Read the model definition and answer for the solid it produces. Units are mm, in the model's axes. Round coordinates to 2 decimals unless told otherwise and drop trailing zeros. Order: outer loops, then holes, each group sorted by start corner. A loop starts at its lowest first (then second) coordinate and runs counter-clockwise, first axis right, second up.
from build123d import *
from OCP.BRepFilletAPI import BRepFilletAPI_MakeChamfer

# Parameters (mm, degrees)
SKETCH2_R           = 49.911
SKETCH2_R_2         = 7.62
SKETCH2_R_3         = 9.6266
BOSS_EXTRUDE3_DEPTH = 7.62
SKETCH4_R           = 4.064
CUT_EXTRUDE1_DEPTH  = 71.994931101
SKETCH5_R           = 1.905
SKETCH5_R_2         = 9.6266
CUT_EXTRUDE2_DEPTH  = 71.994931101
CHAMFER1_SIZE       = 2.032
CHAMFER1_SIZE2      = 1.422821718


with BuildPart() as part:
    # Sketch2 → Boss-Extrude3 (new body)
    with BuildSketch(Plane.XY):
        with Locations(Location((0, 0, 0), (0, 0, 180))):
            Circle(SKETCH2_R)
        with Locations(Location((0, 0, 0), (0, 0, 180))):
            Circle(SKETCH2_R_2, mode=Mode.SUBTRACT)
        with Locations(Location((0.005302646, -19.066344944, 0), (0, 0, 180))):
            Circle(SKETCH2_R_3, mode=Mode.SUBTRACT)
        with Locations(Location((18.140112855, -5.903126437, 0), (0, 0, 180))):
            Circle(SKETCH2_R_3, mode=Mode.SUBTRACT)
        with Locations(Location((11.225112662, 15.411761203, 0), (0, 0, 180))):
            Circle(SKETCH2_R_3, mode=Mode.SUBTRACT)
        with Locations(Location((-11.183402698, 15.421867724, 0), (0, 0, 180))):
            Circle(SKETCH2_R_3, mode=Mode.SUBTRACT)
        with Locations(Location((-18.117626635, -5.886773743, 0), (0, 0, 180))):
            Circle(SKETCH2_R_3, mode=Mode.SUBTRACT)
        with Locations(Location((-38.862, 0, 0), (0, 0, 180))):
            Circle(SKETCH2_R_3, mode=Mode.SUBTRACT)
        with Locations(Location((-31.453761301, -22.864504732, 0), (0, 0, 180))):
            Circle(SKETCH2_R_3, mode=Mode.SUBTRACT)
        with Locations(Location((-12.020951612, -37.007824175, 0), (0, 0, 180))):
            Circle(SKETCH2_R_3, mode=Mode.SUBTRACT)
        with Locations(Location((12.013756262, -37.027691016, 0), (0, 0, 180))):
            Circle(SKETCH2_R_3, mode=Mode.SUBTRACT)
        with Locations(Location((31.469920822, -22.916516796, 0), (0, 0, 180))):
            Circle(SKETCH2_R_3, mode=Mode.SUBTRACT)
        with Locations(Location((38.915948498, -0.064290447, 0), (0, 0, 180))):
            Circle(SKETCH2_R_3, mode=Mode.SUBTRACT)
        with Locations(Location((31.507709799, 22.800214285, 0), (0, 0, 180))):
            Circle(SKETCH2_R_3, mode=Mode.SUBTRACT)
        with Locations(Location((12.07490011, 36.943533728, 0), (0, 0, 180))):
            Circle(SKETCH2_R_3, mode=Mode.SUBTRACT)
        with Locations(Location((-11.959807763, 36.963400568, 0), (0, 0, 180))):
            Circle(SKETCH2_R_3, mode=Mode.SUBTRACT)
        with Locations(Location((-31.415972324, 22.852226349, 0), (0, 0, 180))):
            Circle(SKETCH2_R_3, mode=Mode.SUBTRACT)
    extrude(amount=BOSS_EXTRUDE3_DEPTH)

    # Sketch4 → Cut-Extrude1 (cut, through all)
    with BuildSketch(Plane.XY.offset(7.62)):
        with Locations((0, 26.17695394)):
            Circle(SKETCH4_R)
        with Locations((24.895762621, 8.037987129)):
            Circle(SKETCH4_R)
        with Locations((15.337793775, -21.244539145)):
            Circle(SKETCH4_R)
        with Locations((-15.465118457, -21.203168848)):
            Circle(SKETCH4_R)
        with Locations((-24.944396322, 8.104925676)):
            Circle(SKETCH4_R)
    extrude(amount=-CUT_EXTRUDE1_DEPTH, mode=Mode.SUBTRACT)

    # Sketch5 → Cut-Extrude2 (cut, through all)
    with BuildSketch(Plane(origin=(0, 0, 0), x_dir=(-1, 0, 0), z_dir=(0, 0, -1))):
        with Locations((-0.00287222, -45.643800189)):
            Circle(SKETCH5_R)
        with Locations((-0.00287222, -32.960144289)):
            Circle(SKETCH5_R)
        with Locations((12.020951612, -37.007824175)):
            Circle(SKETCH5_R_2)
        with Locations((-43.398142788, -14.092845642)):
            Circle(SKETCH5_R)
        with Locations((-31.335269193, -10.173380418)):
            Circle(SKETCH5_R)
        with Locations((-26.801277951, 36.928290351)):
            Circle(SKETCH5_R)
        with Locations((-19.346012068, 26.666997177)):
            Circle(SKETCH5_R)
        with Locations((26.851419192, 36.910131993)):
            Circle(SKETCH5_R)
        with Locations((19.396153308, 26.648838818)):
            Circle(SKETCH5_R)
        with Locations((43.413744778, -14.122226483)):
            Circle(SKETCH5_R)
        with Locations((31.350871183, -10.20276126)):
            Circle(SKETCH5_R)
    extrude(amount=-CUT_EXTRUDE2_DEPTH, mode=Mode.SUBTRACT)

    # Chamfer1: one chamfer whose edges measure the first distance from different faces: ONE call of the kernel's chamfer builder (chamfer() names one face for all edges)
    chamfer1_edges_1 = [part.edges().sort_by_distance(p)[0] for p in [
        (-4.064, 26.17695394, 0),
    ]]
    chamfer1_side_1 = [part.faces().sort_by_distance(p)[0] for p in [
        (-4.064, 26.17695394, 3.81),
    ]]
    chamfer1_edges_2 = [part.edges().sort_by_distance(p)[0] for p in [
        (20.831762621, 8.037987129, 0),
    ]]
    chamfer1_side_2 = [part.faces().sort_by_distance(p)[0] for p in [
        (20.831762621, 8.037987129, 3.81),
    ]]
    chamfer1_edges_3 = [part.edges().sort_by_distance(p)[0] for p in [
        (11.273793775, -21.244539145, 0),
    ]]
    chamfer1_side_3 = [part.faces().sort_by_distance(p)[0] for p in [
        (11.273793775, -21.244539145, 3.81),
    ]]
    chamfer1_edges_4 = [part.edges().sort_by_distance(p)[0] for p in [
        (-19.529118457, -21.203168848, 0),
    ]]
    chamfer1_side_4 = [part.faces().sort_by_distance(p)[0] for p in [
        (-19.529118457, -21.203168848, 3.81),
    ]]
    chamfer1_edges_5 = [part.edges().sort_by_distance(p)[0] for p in [
        (-29.008396322, 8.104925676, 0),
    ]]
    chamfer1_side_5 = [part.faces().sort_by_distance(p)[0] for p in [
        (-29.008396322, 8.104925676, 3.81),
    ]]
    chamfer1 = BRepFilletAPI_MakeChamfer(part.part.solid().wrapped)
    for e in chamfer1_edges_1:
        chamfer1.Add(CHAMFER1_SIZE, CHAMFER1_SIZE2, e.wrapped, chamfer1_side_1[0].wrapped)  # the first distance lies on this face
    for e in chamfer1_edges_2:
        chamfer1.Add(CHAMFER1_SIZE, CHAMFER1_SIZE2, e.wrapped, chamfer1_side_2[0].wrapped)  # the first distance lies on this face
    for e in chamfer1_edges_3:
        chamfer1.Add(CHAMFER1_SIZE, CHAMFER1_SIZE2, e.wrapped, chamfer1_side_3[0].wrapped)  # the first distance lies on this face
    for e in chamfer1_edges_4:
        chamfer1.Add(CHAMFER1_SIZE, CHAMFER1_SIZE2, e.wrapped, chamfer1_side_4[0].wrapped)  # the first distance lies on this face
    for e in chamfer1_edges_5:
        chamfer1.Add(CHAMFER1_SIZE, CHAMFER1_SIZE2, e.wrapped, chamfer1_side_5[0].wrapped)  # the first distance lies on this face
    add(Compound.cast(chamfer1.Shape()), mode=Mode.REPLACE)


solid = part.part
Q1. Flat-ended cylindrical pins translate along their axes: pin 1 (17.5 mm diameter, centred on x = 31.51, y = 22.8, fed in from +Z); pin 2 (1 mm diameter, centred on x = 25.5, z = 2, fed in from -Y); pin 3 (2 mm diameter, centred on x = 5, z = 1.5, fed in from -Y); pin 4 (3 mm diameter, centred on x = -3, y = 28, fed in from -Z). Find the tip coordinate at first contact, or state that the pin passes through.
Outcome:
pin 1: passes through
pin 2: stops at y = -43.2
pin 3: stops at y = -49.75
pin 4: stops at z = 0.68
Q2. Straight lines are drawn through the part: probe 1 along X at (y, z) = (27, 4.5); probe 2 along X at (y, z) = (24, 0.5); probe 3 along X at (y, z) = (-30, 2). For each, find the intervals that lie inside material, in ascending order.
Outcome:
probe 1: x = -41.98 to -40.1, -22.73 to -21.27, -17.52 to -3.98, 3.98 to 17.47, 21.22 to 22.85, 40.17 to 41.98
probe 2: x = -43.76 to -40.97, -21.86 to -15.55, -6.81 to -4.65, 4.65 to 6.88, 15.57 to 21.96, 41.06 to 43.76
probe 3: x = -39.89 to -37.92, -24.99 to -18.62, -5.42 to 5.43, 18.59 to 24.95, 37.99 to 39.89
Q3. For a pull along Y with two mould halves and no side action, classify faces 1 (the face through (8, 3, 7.62)), 2 (the face through (19.653, -31.17, 3.757)) as released by +Y, released by -Y, zero draft, split by the parting line, or undercut.
Outcome:
face 1: zero draft
face 2: undercut
Q4. A cutting plane is placed at B-B, the plane x = -32. Give the vertices of the cut face in (y, z).
Outcome:
outline: (-38.3, 0) - (-32.48, 0) - (-32.48, 7.62) - (-38.3, 7.62) - close; (-13.25, 0) - (-11.99, 0) - (-11.99, 7.62) - (-13.25, 7.62) - close; (-8.41, 0) - (-6.75, 0) - (-6.75, 7.62) - (-8.41, 7.62) - close; (6.75, 0) - (13.24, 0) - (13.24, 7.62) - (6.75, 7.62) - close; (32.46, 0) - (38.3, 0) - (38.3, 7.62) - (32.46, 7.62) - close
Q5. A cutting plane is placed at A-A, the plane x = 0. Give the vertices of the cut face in (y, z), plus the area to 3 significant figures.
Outcome:
outline: (-49.91, 0) - (-47.55, 0) - (-47.55, 7.62) - (-49.91, 7.62) - close; (-43.74, 0) - (-34.87, 0) - (-34.87, 7.62) - (-43.74, 7.62) - close; (-31.06, 0) - (-28.69, 0) - (-28.69, 7.62) - (-31.06, 7.62) - close; (-9.44, 0) - (-7.62, 0) - (-7.62, 7.62) - (-9.44, 7.62) - close; (7.62, 0) - (20.69, 0) - (22.11, 2.03) - (22.11, 7.62) - (7.62, 7.62) - close; (30.24, 2.03) - (31.66, 0) - (49.91, 0) - (49.91, 7.62) - (30.24, 7.62) - close
area: 375 mm2
Q6. A cutting plane is placed at C-C, the plane z = 4.5. Give the number of separate pieces and of enclosed holes in the cut face, plus the area to 3 significant figures.
Outcome:
separate pieces: 1
enclosed holes: 31
area: 2,900 mm2
